from build123d import *

# Parameters (mm, degrees)
F0_R     = 180
F0_R_2   = 10
F1_DEPTH = 25
F2_R     = 130
F3_DEPTH = 5
F4_R     = 120
F5_DEPTH = 30.001


with BuildPart() as f1:
    # F0 (on Top) → F1 (new body)
    with BuildSketch(Plane.XY):
        Circle(F0_R)
        with Locations((-115.094368, -111.145339)):
            Circle(F0_R_2, mode=Mode.SUBTRACT)
        with Locations((-75.11545, -141.271615)):
            Circle(F0_R_2, mode=Mode.SUBTRACT)
        with Locations((-27.783708, -157.56924)):
            Circle(F0_R_2, mode=Mode.SUBTRACT)
        with Locations((-143.807047, -70.139383)):
            Circle(F0_R_2, mode=Mode.SUBTRACT)
        with Locations((-158.442891, -22.267696)):
            Circle(F0_R_2, mode=Mode.SUBTRACT)
        with Locations((22.267696, -158.442891)):
            Circle(F0_R_2, mode=Mode.SUBTRACT)
        with Locations((70.139383, -143.807047)):
            Circle(F0_R_2, mode=Mode.SUBTRACT)
        with Locations((111.145339, -115.094368)):
            Circle(F0_R_2, mode=Mode.SUBTRACT)
        with Locations((141.271615, -75.11545)):
            Circle(F0_R_2, mode=Mode.SUBTRACT)
        with Locations((157.56924, -27.783708)):
            Circle(F0_R_2, mode=Mode.SUBTRACT)
        with Locations((-157.56924, 27.783708)):
            Circle(F0_R_2, mode=Mode.SUBTRACT)
        with Locations((-141.271615, 75.11545)):
            Circle(F0_R_2, mode=Mode.SUBTRACT)
        with Locations((-111.145339, 115.094368)):
            Circle(F0_R_2, mode=Mode.SUBTRACT)
        with Locations((-70.139383, 143.807047)):
            Circle(F0_R_2, mode=Mode.SUBTRACT)
        with Locations((-22.267696, 158.442891)):
            Circle(F0_R_2, mode=Mode.SUBTRACT)
        with Locations((158.442891, 22.267696)):
            Circle(F0_R_2, mode=Mode.SUBTRACT)
        with Locations((143.807047, 70.139383)):
            Circle(F0_R_2, mode=Mode.SUBTRACT)
        with Locations((27.783708, 157.56924)):
            Circle(F0_R_2, mode=Mode.SUBTRACT)
        with Locations((75.11545, 141.271615)):
            Circle(F0_R_2, mode=Mode.SUBTRACT)
        with Locations((115.094368, 111.145339)):
            Circle(F0_R_2, mode=Mode.SUBTRACT)
    extrude(amount=F1_DEPTH)

    # F2 (on face) → F3 (join)
    with BuildSketch(Plane.XY.offset(25)):
        Circle(F2_R)
    extrude(amount=F3_DEPTH)

    # F4 (on face) → F5 (cut, through all)
    with BuildSketch(Plane.XY.offset(30)):
        Circle(F4_R)
    extrude(amount=-F5_DEPTH, mode=Mode.SUBTRACT)


solid = f1.part
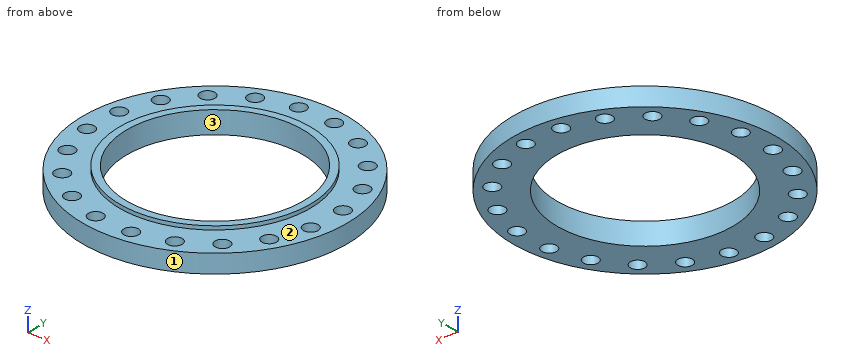
The listing builds one solid part. Answer for the finished solid, in the listing's coordinates (mm). Face numbers are marked on the shaded views. Give positions to 0.01 mm unless a question says otherwise; leave off trailing zeros. Write each loop counter-clockwise with the first axis right and the second up, starting at its lowest first coordinate (ties: lowest second). Pieces come first, ordered by that corner, then holes.
Item 1: Flat-ended cylindrical pins translate along their axes: P1, Ø16, axis at x = 157.57, y = -27.78, coming from the -Z side; P2, Ø6, axis at y = 40, z = 17.5, coming from the +X side; P3, Ø4, axis at x = 132.5, z = 11.5, coming from the +Y side; P4, Ø1.5, axis at x = 138, z = 11.5, coming from the -Y side. Find the tip coordinate at first contact, or state that the pin passes through.
Item 2: Find the intervals of material crossed by line 1 along X through (y, z) = (19, 4); line 2 along Y through (x, z) = (161.5, 18); line 3 along X through (y, z) = (-162, 15.25), in increasing order.
Item 3: Determine the mould class of the marked faces 1, 2 and 3 for opening direction X: released by +X, released by -X, zero draft, split by the parting line, or undercut.
Item 4: Section C-C, the plane z = 19 is taken. Count the separate pieces of the cut face and the enclosed holes in it, plus the area to 3 significant figures.
Item 5: Section A-A, the plane y = 0 is taken. Write down the section's boundary in (x, z), plus the area to 3 significant figures.
Completed:
1. P1: passes through
1. P2: stops at x = 176.16
1. P3: stops at y = 123.97
1. P4: stops at y = -116.46
2. line 1: x = -178.99 to -162.35, -152.79 to -118.49, 118.49 to 148.99, 167.89 to 178.99
2. line 2: y = -79.48 to -36.98, -18.59 to 12.75, 31.79 to 79.48
2. line 3: x = -78.46 to -36.75, -18.82 to 12.92, 31.61 to 78.46
3. face 1: split by the parting line
3. face 2: zero draft
3. face 3: undercut
4. separate pieces: 1
4. enclosed holes: 21
4. area: 50,300 mm2
5. outline: (-180, 0) - (-120, 0) - (-120, 30) - (-130, 30) - (-130, 25) - (-180, 25) - close; (120, 0) - (180, 0) - (180, 25) - (130, 25) - (130, 30) - (120, 30) - close
5. area: 3,100 mm2
